Read the model definition and answer for the solid it produces. Units are mm, in the model's axes. Coordinates: 2 decimals unless noted, no trailing zeros. Order: outer loops, then holes, each group sorted by start corner. A loop starts at its lowest first (then second) coordinate and runs counter-clockwise, first axis right, second up. Notation, with made-up numbers: M 55,-4.5 L 96,-4.5 A20 cw 96,33.5 Z; hole C 55.5,36 d11. An arc over 180 degrees is marked long. Use a Markdown table: item, result. Add a question column.
1) Find section C-C on z = 4.75. Count the separate pieces of the cut face and the enclosed holes in it, plus the area to 3 significant figures.
2) Find the intervals of material crossed by probe 1 along X at (y, z) = (0.5, 3.25); probe 2 along Y at (x, z) = (-3.25, 20.5); probe 3 along Y at (x, z) = (2, 22.25), in increasing order. Write a range as [from, to].
3) Find section D-D on x = -7. Write down the section's boundary in (y, z), plus the area to 3 significant figures.
4) Each of these flat-tipped pins is pushed along its axis until it touches: pin 1 Ø3 at (x, z) = (-8, 12) entering from -Y; pin 2 Ø1.5 at (y, z) = (-1.5, 8.5) entering from +X; pin 3 Ø6 at (y, z) = (35.5, 10.5) entering from -X; pin 4 Ø11.5 at (x, y) = (0, 0) entering from -Z. Where does it stop, or does it pass through?
5) Find section A-A on x = 0. Write down the section's boundary in (y, z) (3 decimals), plus the area to 3 significant figures.
6) The mould has two halves that part along X. Classify faces 1 (the face through (0.16, 44.45, 12.52)), 2 (the face through (-1.032, 31.863, 12.522)), 3 (the face through (10.264, 19.351, 12.522)): released by +X, released by -X, zero draft, split by the parting line, or undercut.
7) Find section B-B on y = 3. Write down the section's boundary in (x, z), plus the area to 3 significant figures.
from build123d import *

# Parameters (mm, degrees)
F0_R     = 9.525
F0_R_2   = 4.7625
F1_DEPTH = 25.4


with BuildPart() as f1:
    # F0 (on Top) → F1 (new body)
    with BuildSketch(Plane.XY):
        with BuildLine():
            ThreePointArc((-12.591503, 1.656522), (-0.830036, -12.672847), (12.7, 0))
            ThreePointArc((12.7, 0), (12.672847, 0.830036), (12.591503, 1.656522))
            ThreePointArc((12.591503, 1.656522), (0, 12.7), (-12.591503, 1.656522))
        make_face()
        Circle(F0_R, mode=Mode.SUBTRACT)
        with BuildLine():
            ThreePointArc((-12.591503, 1.656522), (0, 12.7), (12.591503, 1.656522))
            Line((12.591503, 1.656522), (7.869689, 37.547826))
            ThreePointArc((7.869689, 37.547826), (7.920529, 37.031272), (7.9375, 36.5125))
            ThreePointArc((7.9375, 36.5125), (-0.518772, 28.591971), (-7.869689, 37.547826))
            Line((-7.869689, 37.547826), (-12.591503, 1.656522))
        make_face()
        with BuildLine():
            ThreePointArc((7.9375, 36.5125), (7.920529, 37.031272), (7.869689, 37.547826))
            ThreePointArc((7.869689, 37.547826), (0, 44.45), (-7.869689, 37.547826))
            ThreePointArc((-7.869689, 37.547826), (-0.518772, 28.591971), (7.9375, 36.5125))
        make_face()
        with Locations((0, 36.5125)):
            Circle(F0_R_2, mode=Mode.SUBTRACT)
    extrude(amount=F1_DEPTH)


solid = f1.part
Check result:
| question | item | result |
|---|---|---|
| 1 | separate pieces | 1 |
| 1 | enclosed holes | 2 |
| 1 | area | 756 mm2 |
| 2 | probe 1 | x = [-12.69, -9.51], [9.51, 12.69] |
| 2 | probe 2 | y = [-12.28, -8.95], [8.95, 33.03], [39.99, 43.75] |
| 2 | probe 3 | y = [-12.54, -9.31], [9.31, 32.19], [40.83, 44.19] |
| 3 | outline | M -10.6,0 L -6.46,0 L -6.46,25.4 L -10.6,25.4 Z; M 6.46,0 L 40.25,0 L 40.25,25.4 L 6.46,25.4 Z |
| 3 | area | 963 mm2 |
| 4 | pin 1 | stops at y = -10.91 |
| 4 | pin 2 | stops at x = 12.68 |
| 4 | pin 3 | stops at x = -8.53 |
| 4 | pin 4 | passes through |
| 5 | outline | M -12.7,0 L -9.525,0 L -9.525,25.4 L -12.7,25.4 Z; M 9.525,0 L 31.75,0 L 31.75,25.4 L 9.525,25.4 Z; M 41.275,0 L 44.45,0 L 44.45,25.4 L 41.275,25.4 Z |
| 5 | area | 726 mm2 |
| 6 | face 1 | split by the parting line |
| 6 | face 2 | undercut |
| 6 | face 3 | released by +X |
| 7 | outline | M -12.41,0 L -9.04,0 L -9.04,25.4 L -12.41,25.4 Z; M 9.04,0 L 12.41,0 L 12.41,25.4 L 9.04,25.4 Z |
| 7 | area | 171 mm2 |
